Here's the drawing with two shaded views (mm, measured from the low corner). I have some questions. A direction names the side the tool comes from. Coordinates: 2 decimals unless noted, no trailing zeros. Write each loop counter-clockwise with the first axis right and the second up, starting at its lowest first coordinate (ties: lowest second). Pieces come first, ordered by that corner, then holes.
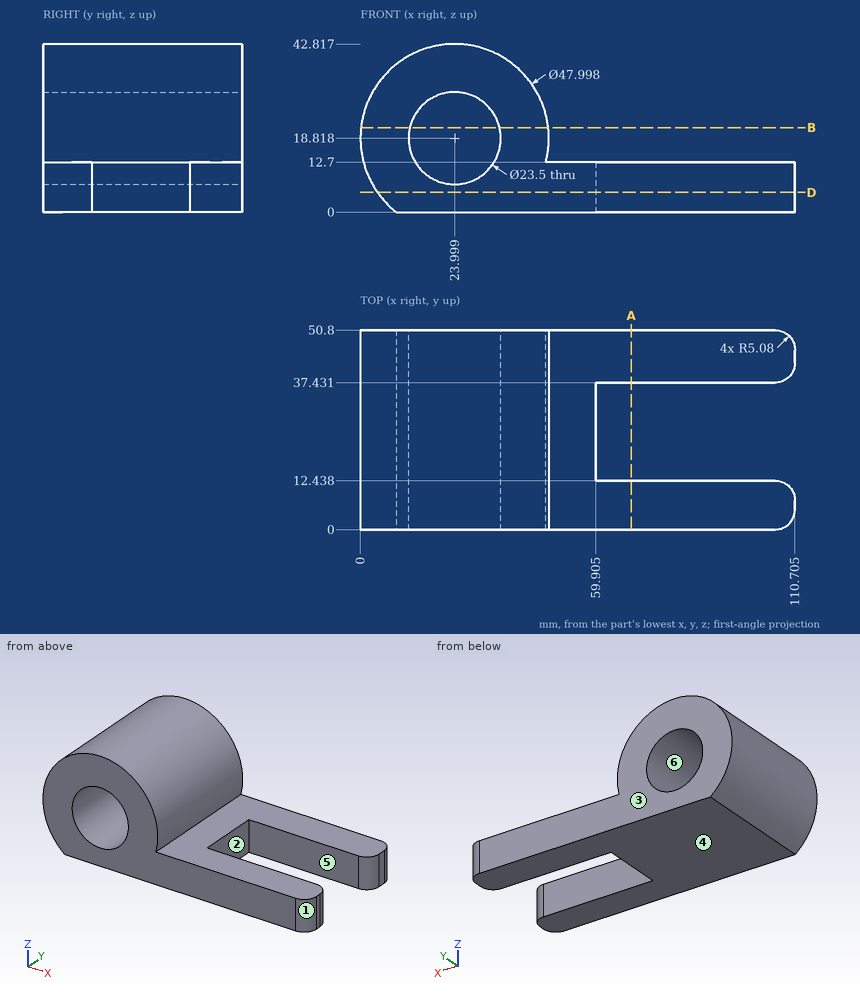
1. For pin 1 (8 mm diameter, centred on x = 81, y = 11, fed in from -Z); pin 2 (12 mm diameter, centred on y = 20.5, z = 32, fed in from -X); pin 3 (3 mm diameter, centred on y = 20.5, z = 4.5, fed in from -X); pin 4 (5 mm diameter, centred on x = 60, y = 5.5, fed in from +Z), each with a flat end and sliding along its axis, tell me the tip position at first contact or that it passes through.
Verdict:
pin 1: stops at z = 0
pin 2: stops at x = 1.1
pin 3: stops at x = 3.71
pin 4: stops at z = 12.7
2. I want a section at A-A on x = 69. Please give me the cut outline in (y, z), plus the area to 3 significant figures.
Verdict:
outline: (0, 0) - (12.44, 0) - (12.44, 12.7) - (0, 12.7) - close; (37.43, 0) - (50.8, 0) - (50.8, 12.7) - (37.43, 12.7) - close
area: 328 mm2
3. On a 3-axis mill with a long thin cutter (end or side, diameter ignored), from which of +Z, -Z, +X, -X, +Y, -Y can I reach the whole of each face in a straight line? I mean the marked faces 5 and 6. Say none if no direction works.
Verdict:
face 5: +Z, -Z, +X
face 6: +Y, -Y
4. Please list where these lines run through material, in increasing order: line 1 along Z through (x, y) = (78.5, 11.5); line 2 along X through (y, z) = (39.5, 26); line 3 along X through (y, z) = (43, 24) (1 decimal).
Verdict:
line 1: z = 0 to 12.7
line 2: x = 1.1 to 14.7, 33.3 to 46.9
line 3: x = 0.6 to 13.5, 34.5 to 47.4
5. If we mould it in two halves opening along Y, with no side actions, what happens to the marked faces 1, 2, 3 and 4? For each: pulls with the +Y half, pulls with the -Y half, needs draft (parallel to the pull), parting line crosses it, or undercut.
Verdict:
face 1: pulls with the -Y half
face 2: undercut
face 3: pulls with the +Y half
face 4: needs draft
6. I want a section at D-D on z = 5. Please give me the cut outline in (x, y) (1 decimal).
Verdict:
outline: (4.4, 0) - (105.6, 0) arc R5.1 ccw to (110.7, 5.1) - (110.7, 7.4) arc R5.1 ccw to (105.6, 12.4) - (59.9, 12.4) - (59.9, 37.4) - (105.6, 37.4) arc R5.1 ccw to (110.7, 42.5) - (110.7, 45.7) arc R5.1 ccw to (105.6, 50.8) - (4.4, 50.8) - close
7. I want a section at B-B on z = 21.5. Please give me the cut outline in (x, y).
Verdict:
outline: (0.15, 0) - (12.56, 0) - (12.56, 50.8) - (0.15, 50.8) - close; (35.44, 0) - (47.85, 0) - (47.85, 50.8) - (35.44, 50.8) - close
